Autodesk Inventor part; units mm, degrees
ref_plane "YZ Plane" through (0, 0, 0) normal (1, 0, 0) x (0, 1, 0)
ref_plane "XZ Plane" through (0, 0, 0) normal (0, 1, 0) x (-1, 0, 0)
ref_plane "XY Plane" through (0, 0, 0) normal (0, 0, 1) x (1, 0, 0)
ref_plane "Plano de trabajo1" through (0, 0, 0) normal (0, 0, 1) x (1, 0, 0)
sketch "Boceto1" plane through (0, 0, 0) normal (0, 0, 1) x (1, 0, 0)
  circle A0 centre (10.9923, 0) radius 10.9823
  circle A1 centre (10.9923, 0) radius 3.1378
  circle A2 centre (18.3423, 0) radius 1.2028
  circle A3 centre (10.9923, 7.35) radius 1.2028
  circle A4 centre (3.6423, 0) radius 1.2028
  circle A5 centre (10.9923, -7.35) radius 1.2028
  line L0 (0, 0) -> (0, 30)
  line L1 (21.9746, 0) -> (21.9746, -30)
  line L2 (0, 0) -> (0, -30)
  line L3 (0, -30) -> (21.9746, -30)
  circle A6 centre (10.9923, 0) radius 3.1378
  circle A7 centre (18.3423, 0) radius 1.2028
  circle A8 centre (10.9923, -7.35) radius 1.2028
  circle A9 centre (3.6423, 0) radius 1.2028
  circle A10 centre (10.9923, 7.35) radius 1.2028
  circle A11 centre (10.9923, 0) radius 10.9823
  line L4 (0, 0) -> (0, -30)
  line L5 (0, -30) -> (21.9746, -30)
  line L6 (21.9746, -30) -> (21.9746, 0)
  dimension "d0" = 30
  dimension "d1" = 30
extrude "Extrusión1" add sketch "Boceto1" along normal blind 3
sketch "Boceto2" plane through (10.9923, 0, 3) normal (0, 0, 1) x (1, 0, 0)
  circle A0 centre (0, 0) radius 10.9823
  line L0 (10.9823, 0) -> (10.9823, -30)
  line L1 (10.9823, -30) -> (-9.7118, -30)
  line L2 (-9.7118, -30) -> (-10.9923, 0)
  circle A1 centre (0, 0) radius 10.9823
  circle A2 centre (0, -7.35) radius 1.2028
  circle A3 centre (-7.35, 0) radius 1.2028
  circle A4 centre (0, 7.35) radius 1.2028
  circle A5 centre (7.35, 0) radius 1.2028
  circle A6 centre (0, 0) radius 3.1378
  point P0 (-10.9723, -0.4683)
  dimension "d4" = 30
extrude "Extrusión2" add sketch "Boceto2" against normal blind 3 contours L0 L1 L2 A0
sketch "Boceto3" plane through (0, 0, 0) normal (0, 0, -1) x (-1, 0, 0)
  point P0 (0, 0)
sketch "Boceto4" plane through (0, 0, 3) normal (0, 0, 1) x (1, 0, 0)
  point P0 (0, 0)
sketch "Boceto5" plane through (0, 0, 0) normal (0, 0, -1) x (-1, 0, 0)
  arc A0 (-0.02, -0.4683) -> (-21.9746, 0) centre (-10.9923, 0) ccw
  line L0 (-21.9746, 0) -> (-21.9746, -30)
  line L1 (-21.9746, -30) -> (-1.2805, -30)
  line L2 (-1.2805, -30) -> (-0.02, -0.4683)
  circle A1 centre (-10.9923, -7.35) radius 1.2028
  circle A2 centre (-3.6423, 0) radius 1.2028
  circle A3 centre (-10.9923, 7.35) radius 1.2028
  circle A4 centre (-18.3423, 0) radius 1.2028
  circle A5 centre (-10.9923, 0) radius 3.1378
  line L3 (-21.9746, -30) -> (0, -30)
  line L4 (0, -30) -> (0, 0)
  line L5 (0, 0) -> (-21.9746, 0)
  line L6 (-21.9746, 0) -> (-21.9746, -30)
  point P0 (-0.01, 0)
extrude "Extrusión3" add sketch "Boceto5" against normal blind 3 contours A0 L5 L4 L3 L2
sketch "Boceto6" plane through (0, 0, 0) normal (0, 0, -1) x (-1, 0, 0)
  point P0 (0, 0)
sketch "Boceto7" plane through (0, 0, 0) normal (0, 0, -1) x (-1, 0, 0)
  line L0 (-21.9746, -30) -> (0, -30)
  line L1 (-21.9746, -30) -> (-21.9746, 0)
  line L2 (0, -30) -> (-21.9746, -30)
  line L3 (-21.9746, -30) -> (-21.9746, -27)
  line L4 (-21.9746, -27) -> (0, -27)
  line L5 (0, -27) -> (0, -30)
  point P0 (0, 0)
  dimension "d9" = 3
extrude "Extrusión4" add sketch "Boceto7" along normal blind 40
sketch "Boceto8" plane through (0, -27, 0) normal (0, 1, 0) x (1, 0, 0)
  line L0 (0, -3) -> (0, 40)
  line L1 (21.9746, -3) -> (21.9746, 40)
  line L2 (0, 40) -> (21.9746, 40)
  line L3 (21.9746, 40) -> (21.9746, 38)
  line L4 (21.9746, 38) -> (0, 38)
  line L5 (0, 38) -> (0, 40)
  point P0 (0, 0)
  point P1 (21.9746, 40)
  point P2 (0, 38)
  dimension "d12" = 2
extrude "Extrusión5" add sketch "Boceto8" along normal blind 40
sketch "Boceto9" plane through (0, 0, -40) normal (0, 0, -1) x (-1, 0, 0)
  circle A0 centre (-11.0072, -0.015) radius 2.7
  circle A1 centre (-11.0099, -0.0117) radius 10.9823
  circle A2 centre (-18.3423, 0) radius 1.2028
  circle A3 centre (-10.9923, -7.35) radius 1.2028
  circle A4 centre (-10.9923, 7.35) radius 1.2028
  circle A5 centre (-3.6423, 0) radius 1.2028
  line L0 (-21.9746, -30) -> (-21.9746, 13)
  line L1 (-21.9746, -30) -> (0, -30)
  line L2 (0, -30) -> (0, 13)
  line L3 (-21.9746, 13) -> (0, 13)
  line L4 (-21.5706, 0) -> (-25.972, 0)
  line L5 (-25.972, 0) -> (-25.972, 18.1609)
  line L6 (-25.972, 18.1609) -> (4.5124, 18.1609)
  line L7 (4.5124, 18.1609) -> (4.5124, 1.2028)
  line L8 (4.5124, 1.2028) -> (4.5124, 0)
  line L9 (-3.6423, 0) -> (4.822, 0)
  point P0 (0, 0)
  point P1 (-21.9746, 0.6093)
  point P2 (-0.0276, 0)
  point P3 (0, 0)
extrude "Extrusión6" cut sketch "Boceto9" against normal blind 40 contours A0 | A1 L0 L3 L2 L9 | A2 | A3 | A4 | A5
sketch "Boceto10" plane through (0, -30, 3) normal (0, -1, 0) x (1, 0, 0)
  point P0 (0, -3)
sketch "Boceto11" plane through (0, -30, 3) normal (0, -1, 0) x (1, 0, 0)
  line L0 (0.0276, -43) -> (21.9746, -43)
  line L1 (0, -3) -> (0, 0)
  line L2 (21.9746, -43) -> (0, -43)
  line L3 (0, -43) -> (0, 0)
  line L4 (0, 0) -> (21.9746, 0)
  line L5 (21.9746, 0) -> (21.9746, -43)
  line L6 (0, -43) -> (-100, -43)
  line L7 (-100, -43) -> (-100, 0)
  line L8 (-100, 0) -> (0, 0)
  line L9 (0, 0) -> (0, -43)
  line L10 (-100, 0) -> (-100, -21.5)
  line L11 (-100, -21.5) -> (-100, -14.5)
  line L12 (-100, -14.5) -> (-100, -28.5)
  line L13 (-100, -28.5) -> (-50, -43)
  line L14 (-50, -43) -> (-50, 0)
  line L15 (-100, -14.5) -> (-50, 0)
  dimension "d17" = 100
  dimension "d18" = 21.5
  dimension "d19" = 7
  dimension "d20" = 14
extrude "Extrusión7" add sketch "Boceto11" along normal blind 10 contours L2 L3 L1 L4 L5 L0 | L6 L14 L8 L1 L3 | L13 L7 L15 L14
chamfer "Chaflán1" distance 2 angle 45 12 edges at (-14.0127, -40, -40) (-75, -40, -32.75) (-75, -30, -32.75) (-25, -30, -40) (-14.0127, -40, 3) (-75, -40, -4.25) (-100, -40, -18.5) (-75, -30, -4.25) (-25, -30, 3) (-100, -30, -18.5) (-100, -35, -25.5) (-100, -35, -11.5)
sketch "Boceto12" plane through (0, -40, 3) normal (0, -1, 0) x (1, 0, 0)
  line L0 (-49.7159, -2) -> (21.9746, -2)
  line L1 (-98, -16.0024) -> (-49.7159, -2)
  line L2 (-98, -26.9976) -> (-98, -16.0024)
  line L3 (-49.7159, -41) -> (-98, -26.9976)
  line L4 (21.9746, -41) -> (-49.7159, -41)
  line L5 (21.9746, -41) -> (21.9746, -2)
  line L6 (-48.5793, -33) -> (-88.2344, -21.5)
  line L7 (-88.2344, -21.5) -> (-48.5793, -10)
  line L8 (-48.5793, -10) -> (13.9746, -10)
  line L9 (13.9746, -10) -> (13.9746, -33)
  line L10 (13.9746, -33) -> (-48.5793, -33)
  point P0 (0, -3)
  dimension "d26" = 8
extrude "Extrusión8" cut sketch "Boceto12" against normal blind 4 contours L6 L7 L8 L9 L10
sketch "Boceto13" plane through (0, 0, -40) normal (0, 0, -1) x (-1, 0, 0)
  circle A0 centre (-11.0099, -0.0117) radius 5.6
  circle A1 centre (-11.0072, -0.015) radius 2.7
  point P0 (0, 0)
extrude "Extrusión9" cut sketch "Boceto13" against normal blind 5
properties part number "tibia"
Model file for the job. Use its own axes, mm. A direction names the side the tool comes from. Give positions to 0.01 mm unless a question says otherwise; leave off trailing zeros. Order: outer loops, then holes, each group sorted by start corner. A loop starts at its lowest first (then second) coordinate and runs counter-clockwise, first axis right, second up. Notation, with made-up numbers: M 21.5,27.25 L 53.5,27.25 A15 ccw 53.5,36.25 Z; hole C 77.25,75.25 d10. An arc over 180 degrees is marked long. Put each result on its own line as item: value. Start each with the question number.
(1) Tool access for faces 5 (the face through (-17, -38, -30)), 6 (the face through (-99.026, -34.958, -12.204)), 7 (the face through (15.454, -3.419, -39.014)): list every direction of +Z, -Z, +X, -X, +Y, -Y with a clear straight run to the whole face (end or side of a thin tool).
(2) Drill centre lines: L1, parallel to X at y = -29.5, z = -19; L2, parallel to Z at x = 10, y = -11.5; L3, parallel to Y at x = -68, z = -28. Where is each one in solid material? Low to high. Write a range as [from, to].
(3) Band-saw the part on C-C on x = -36.5. Give the cut face in (y, z), then the cut area to 3 significant figures.
(4) Band-saw the part on D-D on z = -2. Give the cut face in (x, y), then the cut area to 3 significant figures.
(5) Pull direction Y, two halves, no side cores. Call faces 1 (the face through (11, -12, 0)), 2 (the face through (17.195, 0.361, -39.014)), 3 (the face through (-74, -39, -32)), 4 (the face through (11.547, -6.283, 1.479)): released by +Y, released by -Y, zero draft, split by the parting line, or undercut.
(6) Band-saw the part on B-B on y = -7.35. Give the cut face in (x, z), then the cut area to 3 significant figures.
(7) Band-saw the part on A-A on y = -13.5. Give the cut face in (x, z), then the cut area to 3 significant figures.
(8) Pin check, flat tips, straight feed: pin 1 Ø2 at (x, y) = (3.64, 0) entering from +Z; pin 2 Ø5 at (x, z) = (-27, -33.5) entering from +Y; pin 3 Ø5 at (x, y) = (-85.5, -29) entering from +Z; pin 4 Ø6 at (x, z) = (-6.5, -18) entering from -Y. Stop position of each tip, or through.
Results below:
1. face 5: -Y
1. face 6: +Z, -X, +Y, -Y
1. face 7: -Z
2. L1: x = [0, 21.97]
2. L2: z = [-40, -38], [0, 3]
2. L3: y = [-40, -30]
3. outline: M -40,-38 L -38,-40 L -32,-40 L -30,-38 L -30,1 L -32,3 L -38,3 L -40,1 L -40,-7 L -36,-7 L -36,-30 L -40,-30 Z
3. area: 330 mm2
4. outline: M -67.24,-38 L -60.06,-40 L 21.97,-40 L 21.97,-27 L 0,-27 L 0,-30 L -60.06,-30 L -67.24,-32 Z
4. area: 944 mm2
5. face 1: zero draft
5. face 2: undercut
5. face 3: released by -Y
5. face 4: undercut
6. outline: M 0,-40 L 9.79,-40 L 9.79,-38 L 0,-38 Z; M 0,0 L 9.79,0 L 9.79,3 L 0,3 Z; M 12.2,-40 L 21.97,-40 L 21.97,-38 L 12.2,-38 Z; M 12.2,0 L 21.97,0 L 21.97,3 L 12.2,3 Z
6. area: 97.8 mm2
7. outline: M 0,-40 L 21.97,-40 L 21.97,-38 L 0,-38 Z; M 0,0 L 21.97,0 L 21.97,3 L 0,3 Z
7. area: 110 mm2
8. pin 1: passes through
8. pin 2: stops at y = -30
8. pin 3: stops at z = -7.72
8. pin 4: stops at y = -36
